Work out the finished part from the listing and answer in its coordinate system (mm). Face numbers are marked on the shaded views. A direction names the side the tool comes from. Round coordinates to 2 decimals unless told otherwise and drop trailing zeros. Loops run counter-clockwise (first coordinate to the right, second up) from the corner with the lowest first, then second, coordinate; pieces in that order, holes last.
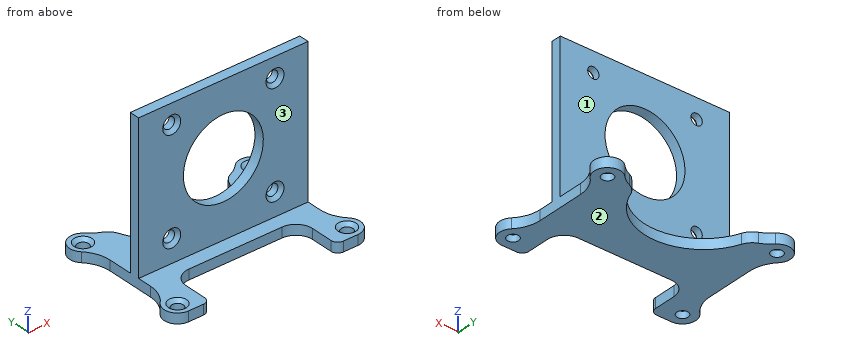
```python
from build123d import *

# Parameters (mm, degrees)
SKETCH_1_R          = 1.7
EXTRUDE_1_DEPTH     = 3
EXTRUDE_2_DEPTH     = 44
SKETCH_3_R          = 1.7
SKETCH_3_R_2        = 12
CUT_EXTRUDE_1_DEPTH = 4
SKETCH_4_W          = 38
SKETCH_4_H          = 9.646779348
SKETCH_4_H_2        = 4
CUT_EXTRUDE_2_DEPTH = 4
FILLET_1_R          = 10
CHAMFER_1_SIZE      = 1
CHAMFER_2_SIZE      = 1
FILLET_4_R          = 5
FILLET_5_R          = 2
FILLET_6_R          = 5


with BuildPart() as part:
    # Эскиз1 → Бобышка-Вытянуть1 (new body)
    with BuildSketch(Plane.XY):
        with BuildLine():
            ThreePointArc((0, 4), (-4, 0), (0, -4))
            Line((0, -4), (50.89, -4))
            ThreePointArc((50.89, -4), (54.89, 0), (50.89, 4))
            Line((50.89, 4), (50.89, 30))
            ThreePointArc((50.89, 30), (53.718427125, 36.828427125), (46.89, 34))
            Line((46.89, 34), (4, 34))
            ThreePointArc((4, 34), (-2.828427125, 36.828427125), (0, 30))
            Line((0, 30), (0, 4))
        make_face()
        with Locations((50.89, 34)):
            Circle(SKETCH_1_R, mode=Mode.SUBTRACT)
        Circle(SKETCH_1_R, mode=Mode.SUBTRACT)
        with Locations((50.89, 0)):
            Circle(SKETCH_1_R, mode=Mode.SUBTRACT)
        with Locations((0, 34)):
            Circle(SKETCH_1_R, mode=Mode.SUBTRACT)
    extrude(amount=EXTRUDE_1_DEPTH)

    # Эскиз2 → Бобышка-Вытянуть2 (add)
    with BuildSketch(Plane.XY.offset(3)):
        Polygon((50.89, 17), (28.893119951, 17), (0, 17), (0, 14), (50.89, 14), align=None)
    extrude(amount=EXTRUDE_2_DEPTH)

    # Эскиз3 → Вырез-Вытянуть1 (cut)
    with BuildSketch(Plane(origin=(0, 17, 0), x_dir=(1, 0, 0), z_dir=(0, 1, 0))):
        with Locations(Location((9.945, -40.999892664, 0), (0, 0, 270))):
            Circle(SKETCH_3_R)
        with Locations(Location((25.445, -25.5, 0), (0, 0, 270))):
            Circle(SKETCH_3_R_2)
        with Locations(Location((9.945, -9.924036406, 0), (0, 0, 270))):
            Circle(SKETCH_3_R)
        with Locations(Location((40.945, -9.924036406, 0), (0, 0, 270))):
            Circle(SKETCH_3_R)
        with Locations(Location((40.945, -40.999892664, 0), (0, 0, 270))):
            Circle(SKETCH_3_R)
    extrude(amount=-CUT_EXTRUDE_1_DEPTH, mode=Mode.SUBTRACT)

    # Эскиз4 → Вырез-Вытянуть2 (cut)
    with BuildSketch(Plane.XY.offset(3)):
        with BuildLine():
            Line((25.445, 34), (10.58125454, 34))
            Line((10.58125454, 34), (8.098408954, 34))
            ThreePointArc((8.098408954, 34), (25.445, 20.270756407), (42.791591046, 34))
            Line((42.791591046, 34), (25.445, 34))
        make_face()
        with Locations((25.445, 4.823389674)):
            Rectangle(SKETCH_4_W, SKETCH_4_H)
        with Locations((25.445, -2)):
            Rectangle(SKETCH_4_W, SKETCH_4_H_2)
    extrude(amount=-CUT_EXTRUDE_2_DEPTH, mode=Mode.SUBTRACT)

    # Скругление1
    # the kernel refuses this fillet: 10 mm, written as the material it adds along each edge
    with BuildSketch(Plane(origin=(0, 30, 0), x_dir=(0, -1, 0), z_dir=(0, 0, 1)), Plane(origin=(50.89, 4, 0), x_dir=(0, 1, 0), z_dir=(0, 0, 1))) as fillet_1_piece_1:
        with BuildLine():
            CenterArc((5.797958971, -10), FILLET_1_R, 90, 44.415308597)
            Line((-1.200583151, -2.857142857), (-1.340553994, -2.714285714))
            ThreePointArc((-1.340553994, -2.714285714), (-0.496723332, -1.472091229), (-0.2, 0))
            Line((-0.2, 0), (0, 0.2))
            Line((0, 0.2), (5.797958971, 0.2))
            Line((5.797958971, 0.2), (5.797958971, 0))
        make_face()
    extrude(amount=3)
    with BuildSketch(Plane(origin=(0, 4, 0), x_dir=(-0.9219149126204018, -0.387392428795552, 0), z_dir=(0, 0, 1)), Plane(origin=(50.89, 30, 0), x_dir=(0.9219149126204016, 0.38739242879555247, 0), z_dir=(0, 0, 1))) as fillet_1_piece_2:
        with BuildLine():
            CenterArc((6.973063718, -9.219149126), FILLET_1_R, 112.792345701, 44.415308597)
            Line((-2.246085408, -5.345224838), (-2.43046839, -5.267746352))
            Line((-2.43046839, -5.267746352), (-0.184382983, 0.077478486))
            Line((-0.184382983, 0.077478486), (0.077478486, 0.184382983))
            ThreePointArc((0.077478486, 0.184382983), (1.549569715, -0.11234035), (3.021660945, 0.184382983))
            Line((3.021660945, 0.184382983), (3.09913943, 0))
        make_face()
    extrude(amount=3)
    with BuildSketch(Plane(origin=(46.89, 34, 0), x_dir=(0.3790827918383792, 0.9253627596418714, 0), z_dir=(0, 0, 1))) as fillet_1_piece_3:
        with BuildLine():
            CenterArc((6.823490253, 9.253627596), FILLET_1_R, 213.100635844, 34.622483912)
            Line((-1.553636308, 3.79251502), (-1.72117884, 3.683292769))
            ThreePointArc((-1.72117884, 3.683292769), (-0.961890706, 1.820440952), (-0.185072552, -0.075816558))
            Line((-0.185072552, -0.075816558), (0.075816558, -0.185072552))
            ThreePointArc((0.075816558, -0.185072552), (1.516331167, 0.098548961), (2.956845776, -0.185072552))
            Line((2.956845776, -0.185072552), (3.032662335, 0))
        make_face()
    extrude(amount=3)
    with BuildSketch(Plane(origin=(4, 34, 0), x_dir=(-0.3790827918383573, 0.9253627596418805, 0), z_dir=(0, 0, 1))) as fillet_1_piece_4:
        with BuildLine():
            CenterArc((6.823490253, -9.253627596), FILLET_1_R, 112.276880243, 34.622483912)
            Line((-1.553636308, -3.79251502), (-1.72117884, -3.683292769))
            ThreePointArc((-1.72117884, -3.683292769), (-0.961890706, -1.820440952), (-0.185072552, 0.075816558))
            Line((-0.185072552, 0.075816558), (0.075816558, 0.185072552))
            ThreePointArc((0.075816558, 0.185072552), (1.516331167, -0.098548961), (2.956845776, 0.185072552))
            Line((2.956845776, 0.185072552), (3.032662335, 0))
        make_face()
    extrude(amount=3)

    # Фаска1
    chamfer_1_edges = [part.edges().sort_by_distance(p)[0] for p in [
        (40.945, 14, 8.224036406),
        (40.945, 14, 39.299892664),
        (9.945, 14, 39.299892664),
        (9.945, 14, 8.224036406),
    ]]
    chamfer(chamfer_1_edges, length=CHAMFER_1_SIZE)

    # Фаска2
    chamfer_2_edges = [part.edges().sort_by_distance(p)[0] for p in [
        (49.19, 34, 3),
        (-1.7, 0, 3),
        (49.19, 0, 3),
        (-1.7, 34, 3),
    ]]
    chamfer(chamfer_2_edges, length=CHAMFER_2_SIZE)

    # Скругление4
    fillet_4_edges = [part.edges().sort_by_distance(p)[0] for p in [
        (6.445, 9.646779348, 1.5),
        (44.445, 9.646779348, 1.5),
    ]]
    fillet(fillet_4_edges, radius=FILLET_4_R)

    # Скругление5
    fillet_5_edges = [part.edges().sort_by_distance(p)[0] for p in [
        (6.445, -4, 1.5),
        (44.445, -4, 1.5),
    ]]
    fillet(fillet_5_edges, radius=FILLET_5_R)

    # Скругление6
    fillet_6_edges = [part.edges().sort_by_distance(p)[0] for p in [
        (8.098408954, 34, 1.5),
        (42.791591046, 34, 1.5),
    ]]
    fillet(fillet_6_edges, radius=FILLET_6_R)


solid = part.part
```
1. Find section B-B (z = 25.5). Write down the section's boundary in (x, y) (3 decimals).
Answer key:
outline: (0, 14) - (13.445, 14) - (13.445, 17) - (0, 17) - close; (37.445, 14) - (50.89, 14) - (50.89, 17) - (37.445, 17) - close
2. Find section D-D (y = 27). Write down the section's boundary in (x, z), then the cut area to 3 significant figures.
Answer key:
outline: (-0.4, 0) - (11.5, 0) - (11.5, 3) - (-0.4, 3) - close; (39.39, 0) - (51.29, 0) - (51.29, 3) - (39.39, 3) - close
area: 71.4 mm2
3. Consider probe 1 along X at (y, z) = (14.9, 25.5) (3 decimals); probe 2 along Y at (x, z) = (34, 15.5); probe 3 along Z at (x, y) = (3, 25). Determine where each line is inside the solid, lowest interval first.
Answer key:
probe 1: x = 0 to 13.445, 37.445 to 50.89
probe 2: y = 14 to 17
probe 3: z = 0 to 3
4. Find section C-C (x = 17). Write down the section's boundary in (y, z), then the cut area to 3 significant figures.
Answer key:
outline: (9.65, 0) - (22.4, 0) - (22.4, 3) - (17, 3) - (17, 16.97) - (14, 16.97) - (14, 3) - (9.65, 3) - close; (14, 34.03) - (17, 34.03) - (17, 47) - (14, 47) - close
area: 119 mm2
5. Which of the six approach directions +Z, -Z, +X, -X, +Y, -Y give full straight-line access (tool end or side, diameter ignored) to the marked faces 1, 2 and 3?
Answer key:
face 1: +Z, +X, -X, +Y
face 2: -Z, +X, -X, +Y, -Y
face 3: +Z, +X, -X, -Y
6. Given pin 1 (4.5 mm diameter, centred on x = 40.94, z = 41, fed in from -Y) (3 decimals); pin 2 (13 mm diameter, centred on x = 20, z = 33, fed in from +Y); pin 3 (12 mm diameter, centred on y = 16, z = 26, fed in from -X), each flat-ended and moving along its own axis, determine where each tip first touches the part or whether it passes through.
Answer key:
pin 1: stops at y = 14.445
pin 2: stops at y = 17
pin 3: stops at x = 0
7. Find section A-A (y = 0). Write down the section's boundary in (x, z) (3 decimals).
Answer key:
outline: (-4, 0) - (-1.7, 0) - (-1.7, 2) - (-2.7, 3) - (-4, 3) - close; (1.7, 0) - (6.445, 0) - (6.445, 3) - (2.7, 3) - (1.7, 2) - close; (44.445, 0) - (49.19, 0) - (49.19, 2) - (48.19, 3) - (44.445, 3) - close; (52.59, 0) - (54.89, 0) - (54.89, 3) - (53.59, 3) - (52.59, 2) - close
